Part print with two shaded views. Sizes in mm from the minimum x, y, z corner. A direction names the side the tool comes from. Coordinates: 2 decimals unless noted, no trailing zeros. Loops run counter-clockwise (first coordinate to the right, second up) from the corner with the lowest first, then second, coordinate; pieces in that order, holes last.
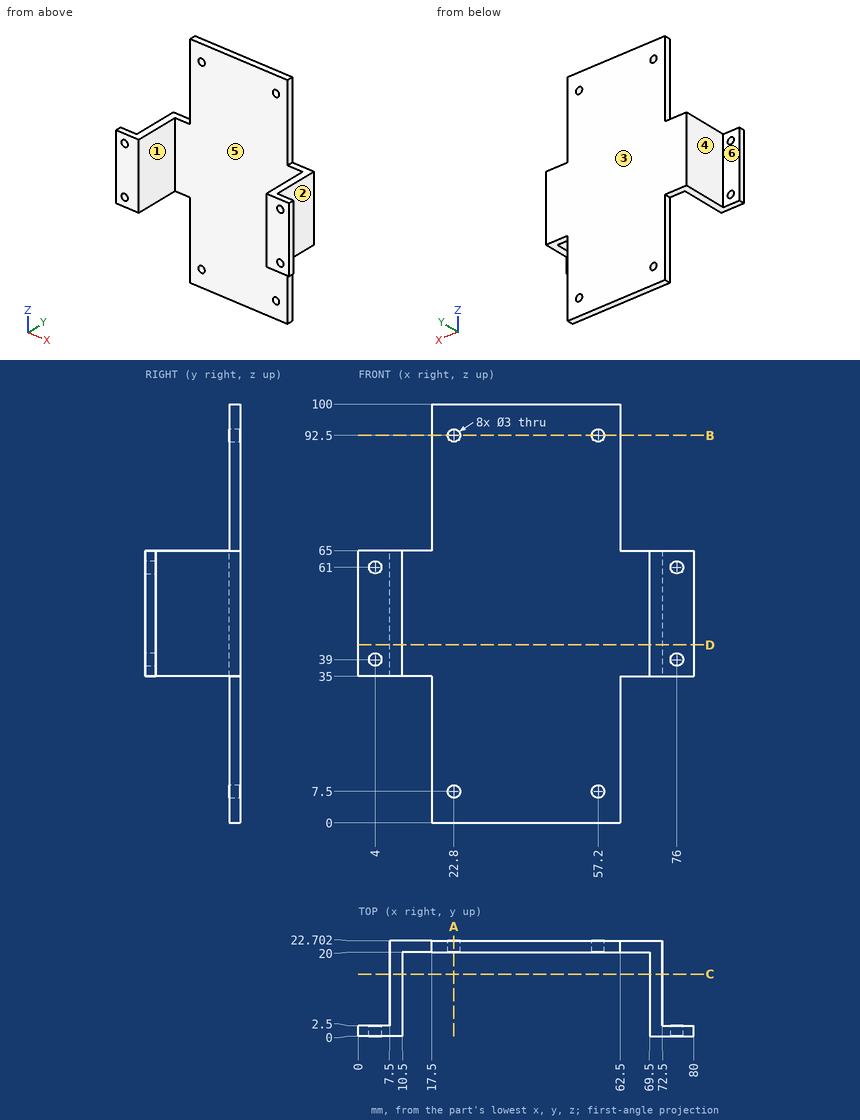
Q1. Slice it at B-B (z = 92.5). List the corners of the cut face in (x, y).
Answers:
outline: (17.5, 20) - (21.3, 20) - (21.3, 22.7) - (17.5, 22.7) - close; (24.3, 20) - (55.7, 20) - (55.7, 22.7) - (24.3, 22.7) - close; (58.7, 20) - (62.5, 20) - (62.5, 22.7) - (58.7, 22.7) - close
Q2. Which spindle directions (+Z, -Z, +X, -X, +Y, -Y) get a long thin tool onto all of the face, cutting with end or side? Do the marked faces 1, 2 and 3. Say none if no direction does.
Answers:
face 1: +Z, -Z, -Y
face 2: +Z, -Z, +X, +Y
face 3: +Z, -Z, +X, -X, +Y
Q3. Mould opens along X. For the marked faces 4, 5 and 6 say: +X half, -X half, draft (parallel to the pull), parting line (faces both ways), or undercut.
Answers:
face 4: -X half
face 5: undercut
face 6: draft
Q4. Slice it at D-D (z = 42.5). List the corners of the cut face in (x, y), and give its area (3 significant figures).
Answers:
outline: (0, 0) - (10.5, 0) - (10.5, 20) - (69.5, 20) - (69.5, 0) - (80, 0) - (80, 2.5) - (72.5, 2.5) - (72.5, 22.7) - (7.5, 22.7) - (7.5, 2.5) - (0, 2.5) - close
area: 333 mm2
Q5. Slice it at C-C (y = 14.75). List the corners of the cut face in (x, z).
Answers:
outline: (7.5, 35) - (10.5, 35) - (10.5, 65) - (7.5, 65) - close; (69.5, 35) - (72.5, 35) - (72.5, 65) - (69.5, 65) - close
Q6. Drill centre lines: line 1 (Z direction, x = 76, y = 1.75); line 2 (X direction, y = 20.95, z = 7.5); line 3 (X direction, y = 0.65, z = 39). Where is each one in solid material? Low to high.
Answers:
line 1: z = 35 to 37.5, 40.5 to 59.5, 62.5 to 65
line 2: x = 17.5 to 21.3, 24.3 to 55.7, 58.7 to 62.5
line 3: x = 0 to 2.5, 5.5 to 10.5, 69.5 to 74.5, 77.5 to 80
Q7. Slice it at A-A (x = 22.8). List the corners of the cut face in (y, z).
Answers:
outline: (20, 0) - (22.7, 0) - (22.7, 6) - (20, 6) - close; (20, 9) - (22.7, 9) - (22.7, 91) - (20, 91) - close; (20, 94) - (22.7, 94) - (22.7, 100) - (20, 100) - close
Q8. Flat gauge pins, fed straight in: P1, Ø2, axis at y = 21.5, z = 10, coming from the -X side; P2, Ø4, axis at x = 75.5, z = 48, coming from the +Y side; P3, Ø9, axis at x = 12.5, y = 14.5, coming from the +Z side. Where does each tip first touch, or does it go through?
Answers:
P1: stops at x = 17.5
P2: stops at y = 2.5
P3: stops at z = 65
